```python
from build123d import *

# Parameters (mm, degrees)
SKETCH_1_R          = 100
EXTRUDE_1_DEPTH     = 70
FILLET_1_R          = 8
SKETCH_2_R          = 5
CUT_EXTRUDE_1_DEPTH = 158.797338444


with BuildPart() as part:
    # 草图1 → 凸台-拉伸1 (new body)
    with BuildSketch(Plane(origin=(0, 0, 0), x_dir=(1, 0, 0), z_dir=(0, 1, 0))):
        with Locations(Location((0, 0, 0), (0, 0, 270))):
            Circle(SKETCH_1_R)
    extrude(amount=EXTRUDE_1_DEPTH)

    # 圆角1
    fillet_1_edges = [part.edges().sort_by_distance(p)[0] for p in [
        (0, 0, -100),
        (0, 70, -100),
    ]]
    fillet(fillet_1_edges, radius=FILLET_1_R)

    # 草图2 → 切除-拉伸1 (cut, through all)
    with BuildSketch(Plane.XZ):
        with Locations(Location((0, 0, 0), (0, 0, 270))):
            Circle(SKETCH_2_R)
    extrude(amount=-CUT_EXTRUDE_1_DEPTH, mode=Mode.SUBTRACT)


solid = part.part
```
The model under review builds one solid part; all positions refer to its coordinate system, in mm. Round coordinates to 2 decimals unless told otherwise and drop trailing zeros. Write each loop counter-clockwise with the first axis right and the second up, starting at its lowest first coordinate (ties: lowest second). Pieces come first, ordered by that corner, then holes.
(1) We need section B-B on x = 0. Give the boundary of the cut face in (y, z), and give its area (3 significant figures).
(2) Wall thickness on L1, parallel to X at y = 15.5, z = 0; L2, parallel to Z at x = -37, y = 65.5; L3, parallel to X at y = 54, z = 39: over which ranges is each line inside the solid? List them lowest first.
(3) Mouldability with a two-part tool opening along Z and no side actions: class faces 1 (the cylindrical face through (-4.88, 34.51, 1.08)), 2 (the cylindrical face through (30.04, 34.62, 95.38)), 3 (the flat face through (1, 70, 19)) as +Z half, -Z half, draft (parallel to the pull), parting line (faces both ways), or undercut.
(4) We need section C-C on y = 41. Give the boundary of the cut face in (x, z).
(5) We need section A-A on z = 0. Give the boundary of the cut face in (x, y).
(6) Insertion check: pin 1 (1 mm diameter, centred on y = 29.5, z = -37.5, fed in from -X); pin 2 (10 mm diameter, centred on x = 7, y = 39.5, fed in from +Z); pin 3 (2 mm diameter, centred on y = 13.5, z = 44, fed in from -X); pin 4 (4 mm diameter, centred on x = 44, z = -13, fed in from -Y). Each pin has a flat end and moves straight along its axis. Give the tip position at first contact, or say it passes through.
Findings below:
1. outline: (0, -92) arc R8 ccw to (8, -100) - (62, -100) arc R8 ccw to (70, -92) - (70, -5) - (0, -5) - close; (0, 5) - (70, 5) - (70, 92) arc R8 ccw to (62, 100) - (8, 100) arc R8 ccw to (0, 92) - close
1. area: 13,200 mm2
2. L1: x = -100 to -5, 5 to 100
2. L2: z = -92.03 to 92.03
2. L3: x = -92.08 to 92.08
3. face 1: undercut
3. face 2: parting line
3. face 3: draft
4. outline: circle Ø200 at (0, 0); hole circle Ø10 at (0, 0)
5. outline: (-100, 8) arc R8 ccw to (-92, 0) - (-5, 0) - (-5, 70) - (-92, 70) arc R8 ccw to (-100, 62) - close; (5, 0) - (92, 0) arc R8 ccw to (100, 8) - (100, 62) arc R8 ccw to (92, 70) - (5, 70) - close
6. pin 1: stops at x = -92.9
6. pin 2: stops at z = 99.98
6. pin 3: stops at x = -90.28
6. pin 4: stops at y = 0
